Check sheet for the modelled part. Datum: model origin and axes. Units: mm. Face numbers are marked on the shaded views. A direction names the side the tool comes from. Give positions to 0.01 mm unless a question says otherwise; leave off trailing zeros. Write each loop counter-clockwise with the first axis right and the second up, starting at its lowest first coordinate (ties: lowest second). Pieces come first, ordered by that corner, then holes. Notation, with made-up numbers: (53.5, 78) -> (106.5, 78) arc R14 cw to (106.5, 90) -> close; hole circle Ø2 at (-7, 58.25). An arc over 180 degrees is marked (long way). Use a Markdown table: item, result. Add a question column.
1. Set-up check for the marked faces 1, 2 and 3: record each of +Z, -Z, +X, -X, +Y, -Y from which the full face is reachable in a straight line by a thin tool's end or side.
2. Cross-section at C-C (z = 21.75). Enter the section's corners in (x, y).
3. Gauge pin test, flat ends, axial feed: P1, Ø3, axis at x = 16, y = 3, coming from the +Z side; P2, Ø8, axis at x = 5.5, y = 8.5, coming from the +Z side; P3, Ø12, axis at x = 23.5, z = 21, coming from the -Y side. Record the tip position at first contact, or that the pin passes through.
4. Cross-section at B-B (z = 15). Enter the section's corners in (x, y), then the cut area to 3 significant figures.
5. Scan lines: probe 1 along Z at (x, y) = (18.25, 5.75); probe 2 along X at (y, z) = (2, 9); probe 3 along Z at (x, y) = (9.75, 1.75). Record each from-to range of solid material in increasing order. Write a range as [from, to].
6. Cross-section at A-A (x = 16.75). Enter the section's corners in (y, z).
from build123d import *

# Parameters (mm, degrees)
F0_W     = 30
F0_H     = 24
F1_DEPTH = 24
F2_W     = 14
F2_H     = 16
F3_DEPTH = 20
F4_W     = 10
F4_H     = 8
F5_DEPTH = 14


with BuildPart() as f1:
    # F0 (on Top) → F1 (new body)
    with BuildSketch(Plane.XY):
        with Locations((15, 12)):
            Rectangle(F0_W, F0_H)
    extrude(amount=F1_DEPTH)

    # F2 (on face) → F3 (cut)
    with BuildSketch(Plane.YZ.offset(30)):
        with Locations((7, 16)):
            Rectangle(F2_W, F2_H)
    extrude(amount=-F3_DEPTH, mode=Mode.SUBTRACT)

    # F4 (on face) → F5 (cut)
    with BuildSketch(Plane.XZ):
        with Locations((5, 20)):
            Rectangle(F4_W, F4_H)
    extrude(amount=-F5_DEPTH, mode=Mode.SUBTRACT)


solid = f1.part
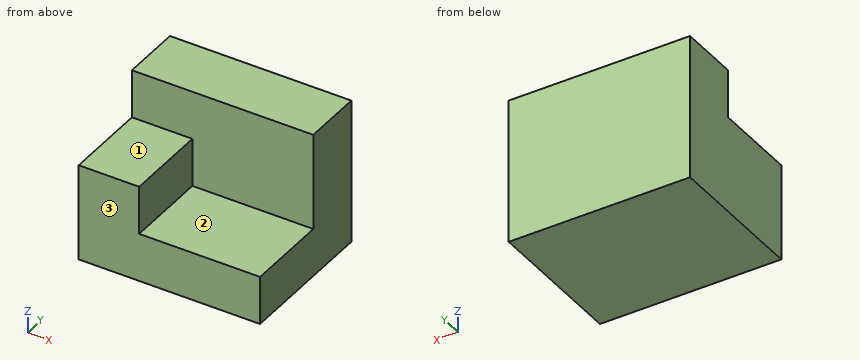
Worked answers:
| question | item | result |
|---|---|---|
| 1 | face 1 | +Z, +X, -X, -Y |
| 1 | face 2 | +Z, +X, -Y |
| 1 | face 3 | +Z, -Z, +X, -X, -Y |
| 2 | outline | (0, 14) -> (30, 14) -> (30, 24) -> (0, 24) -> close |
| 3 | P1 | stops at z = 8 |
| 3 | P2 | stops at z = 16 |
| 3 | P3 | stops at y = 14 |
| 4 | outline | (0, 0) -> (10, 0) -> (10, 14) -> (30, 14) -> (30, 24) -> (0, 24) -> close |
| 4 | area | 440 mm² |
| 5 | probe 1 | z = [0, 8] |
| 5 | probe 2 | x = [0, 10] |
| 5 | probe 3 | z = [0, 16] |
| 6 | outline | (0, 0) -> (24, 0) -> (24, 24) -> (14, 24) -> (14, 8) -> (0, 8) -> close |
